Geometry check sheet. Reference: the model listing, model coordinates, mm. A direction names the side the tool comes from. Round coordinates to 2 decimals unless told otherwise and drop trailing zeros. Order: outer loops, then holes, each group sorted by start corner. A loop starts at its lowest first (then second) coordinate and runs counter-clockwise, first axis right, second up.
Autodesk Inventor part; units mm, degrees
ref_plane "YZ Plane" through (0, 0, 0) normal (1, 0, 0) x (0, 1, 0)
ref_plane "XZ Plane" through (0, 0, 0) normal (0, 1, 0) x (-1, 0, 0)
ref_plane "XY Plane" through (0, 0, 0) normal (0, 0, 1) x (1, 0, 0)
sketch "Sketch1" plane through (0, 0, 0) normal (0, 1, 0) x (-1, 0, 0)
  line L0 (0, 0) -> (-134.62, 0)
  line L1 (-134.62, 0) -> (-134.62, -16.51)
  line L2 (-134.62, -16.51) -> (0, -16.51)
  line L3 (0, -16.51) -> (0, 0)
  line L4 (-134.62, -8.255) -> (-118.11, -8.255)
  line L5 (-118.11, -8.255) -> (-87.63, -8.255)
  line L6 (-87.63, -8.255) -> (-71.12, -8.255)
  line L7 (-71.12, -8.255) -> (-40.64, -8.255)
  line L8 (-40.64, -8.255) -> (-40.64, -122.555)
  line L9 (-40.64, -122.555) -> (-71.12, -122.555)
  line L10 (-71.12, -122.555) -> (-71.12, -8.255)
  line L11 (-87.63, -8.255) -> (-87.63, -122.555)
  line L12 (-87.63, -122.555) -> (-118.11, -122.555)
  line L13 (-118.11, -122.555) -> (-118.11, -8.255)
  line L14 (-118.11, -8.255) -> (-118.11, 106.045)
  line L15 (-118.11, 106.045) -> (-87.63, 106.045)
  line L16 (-87.63, 106.045) -> (-87.63, -8.255)
  line L17 (-71.12, -8.255) -> (-71.12, 106.045)
  line L18 (-71.12, 106.045) -> (-40.64, 106.045)
  line L19 (-40.64, 106.045) -> (-40.64, -8.255)
  dimension "d0" = 134.62
  dimension "d1" = 16.51
  dimension "d2" = 16.51
  dimension "d3" = 30.48
  dimension "d4" = 16.51
  dimension "d5" = 30.48
  dimension "d7" = 114.3
  dimension "d8" = 30.48
  dimension "d9" = 114.3
  dimension "d10" = 30.48
  dimension "d11" = 114.3
  dimension "d12" = 30.48
  dimension "d13" = 114.3
  dimension "d14" = 30.48
extrude "Extrusion1" add sketch "Sketch1" along normal blind 5.08
fillet "Fillet1" radius 5.08 7 edges at (40.64, 2.54, -122.555) (71.12, 2.54, -122.555) (87.63, 2.54, -122.555) (118.11, 2.54, -122.555) (40.64, 2.54, 106.045) (87.63, 2.54, 106.045) (134.62, 2.54, -16.51)
fillet "Fillet2" radius 5.08 3 edges at (71.12, 2.54, 106.045) (118.11, 2.54, 106.045) (134.62, 2.54, 0)
sketch "Sketch2" plane through (0, 5.08, 0) normal (0, 1, 0) x (1, 0, 0)
  line L0 (40.64, 16.51) -> (0, 16.51)
  line L1 (0, 0) -> (8.128, 0)
  line L2 (8.128, 0) -> (8.128, 16.51)
  line L3 (8.128, 16.51) -> (0, 16.51)
  line L4 (0, 16.51) -> (0, 0)
  dimension "d19" = 8.128
extrude "Extrusion2" cut sketch "Sketch2" against normal blind 3.81
sketch "Sketch3" plane through (0, 1.27, 0) normal (0, 1, 0) x (1, 0, 0)
  line L0 (0, 16.51) -> (0, 0)
  line L1 (0, 8.255) -> (3.81, 8.255)
  circle A0 centre (3.81, 8.255) radius 1.397
  line L2 (3.81, 0) -> (3.81, 3.81)
  line L3 (3.81, 16.51) -> (3.81, 12.7)
  circle A1 centre (3.81, 12.7) radius 1.016
  circle A2 centre (3.81, 3.81) radius 1.016
  dimension "d22" = 3.81
  dimension "d23" = 2.794
  dimension "d24" = 3.81
  dimension "d25" = 3.81
  dimension "d26" = 2.032
  dimension "d27" = 2.032
extrude "Extrusion3" cut sketch "Sketch3" against normal blind 1.27
properties part number "Grab Holder v1"
(1) Sectioned sample at A-A, the plane z = 11.5. Record the cut outline in (x, y), and give its area (3 significant figures).
Returned:
outline: (40.64, 0) - (71.12, 0) - (71.12, 5.08) - (40.64, 5.08) - close; (87.63, 0) - (118.11, 0) - (118.11, 5.08) - (87.63, 5.08) - close
area: 310 mm2
(2) Material ranges on line 1 (Z direction, x = 3.81, y = 0.4); line 2 (X direction, y = 1, z = -40); line 3 (Z direction, x = 17, y = 1.75), recorded low to high.
Returned:
line 1: z = -16.51 to -13.72, -11.68 to -9.65, -6.86 to -4.83, -2.79 to 0
line 2: x = 40.64 to 71.12, 87.63 to 118.11
line 3: z = -16.51 to 0
(3) Draft check along X on faces 1 (the cylindrical face through (133.092, 2.576, -1.449)), 2 (the flat face through (25, 3, -16.51)), 3 (the cylindrical face through (69.59, 2.58, 104.6)). Enter one of: released by +X, released by -X, zero draft, split by the parting line, or undercut.
Returned:
face 1: released by +X
face 2: zero draft
face 3: undercut
(4) Depth check by flat-ended pin: P1, Ø2.5, axis at y = 3.5, z = 75.5, coming from the -X side; P2, Ø3, axis at x = 41.5, y = 3.5, coming from the +Z side; P3, Ø1.5, axis at x = 70.5, y = 0.5, coming from the -Z side; P4, Ø1.8, axis at x = 3.81, z = -12.7, coming from the -Y side. Enter the tip coordinate at first touch or a pass-through.
Returned:
P1: stops at x = 40.64
P2: stops at z = 105.26
P3: stops at z = -120.95
P4: passes through
(5) Set-up check for faces 4 (the flat face through (124, 3, -16.51)), 5 (the cylindrical face through (69.7, 2.6, -121)), 6 (the flat face through (79, 3, 0)), 7 (the flat face through (124, 3, 0)): record each of +Z, -Z, +X, -X, +Y, -Y from which the full face is reachable in a straight line by a thin tool's end or side.
Returned:
face 4: -Z, +X, +Y, -Y
face 5: -Z, +Y, -Y
face 6: +Z, +Y, -Y
face 7: +Z, +X, +Y, -Y
